from build123d import *

# Parameters (mm, degrees)
SKETCH1_W               = 79.5
SKETCH1_H               = 76
SKETCH1_R               = 4.05
BOSS_EXTRUDE1_DEPTH     = 79.5
SKETCH2_R               = 4.05
CUT_EXTRUDE1_DEPTH      = 79.5
CUT_EXTRUDE2_DEPTH      = 79.5
CUT_EXTRUDE2_DEPTH_BACK = 79.5
CUT_EXTRUDE3_DEPTH      = 79.5
CUT_EXTRUDE3_DEPTH_BACK = 79.5
SKETCH4_W               = 80.771817398
SKETCH4_H               = 76.525441438


with BuildPart() as part:
    # Sketch1 → Boss-Extrude1 (new body)
    with BuildSketch(Plane(origin=(0, 0, 0), x_dir=(1, 0, 0), z_dir=(0, 1, 0))):
        with Locations((39.75, 0)):
            Rectangle(SKETCH1_W, SKETCH1_H)
        with Locations(Location((20, 20, 0), (0, 0, 90))):
            Circle(SKETCH1_R, mode=Mode.SUBTRACT)
        with Locations(Location((60, 20, 0), (0, 0, 90))):
            Circle(SKETCH1_R, mode=Mode.SUBTRACT)
        with Locations(Location((60, -20, 0), (0, 0, 90))):
            Circle(SKETCH1_R, mode=Mode.SUBTRACT)
        with Locations(Location((20, -20, 0), (0, 0, 90))):
            Circle(SKETCH1_R, mode=Mode.SUBTRACT)
    extrude(amount=BOSS_EXTRUDE1_DEPTH)

    # Sketch2 → Cut-Extrude1 (cut)
    with BuildSketch(Plane(origin=(0, 0, 0), x_dir=(0, 0, -1), z_dir=(1, 0, 0))):
        with Locations((-20, 60)):
            Circle(SKETCH2_R)
        with Locations(Location((20, 60, 0), (0, 0, 180))):
            Circle(SKETCH2_R)
        with Locations(Location((20, 20, 0), (0, 0, 180))):
            Circle(SKETCH2_R)
        with Locations((-20, 20)):
            Circle(SKETCH2_R)
    extrude(amount=CUT_EXTRUDE1_DEPTH, mode=Mode.SUBTRACT)

    # Sketch3 → Cut-Extrude2 (cut, two sides: drawn at the far end of the back side and taken through both)
    with BuildSketch(Plane.XY.offset(-CUT_EXTRUDE2_DEPTH_BACK)):
        Polygon((4, 73.843145751), (4, 4), (73.843145751, 4), align=None)
        Polygon((4, 79.5), (79.5, 4), (79.5, 79.5), align=None)
    extrude(amount=CUT_EXTRUDE2_DEPTH + CUT_EXTRUDE2_DEPTH_BACK, mode=Mode.SUBTRACT)

    # Sketch4 → Cut-Extrude3 (cut, two sides: drawn at the far end of the back side and taken through both)
    with BuildSketch(Plane.XY.offset(-CUT_EXTRUDE3_DEPTH_BACK)):
        with Locations((44.385908699, 42.262720719)):
            Rectangle(SKETCH4_W, SKETCH4_H)
    extrude(amount=CUT_EXTRUDE3_DEPTH + CUT_EXTRUDE3_DEPTH_BACK, mode=Mode.SUBTRACT)


solid = part.part
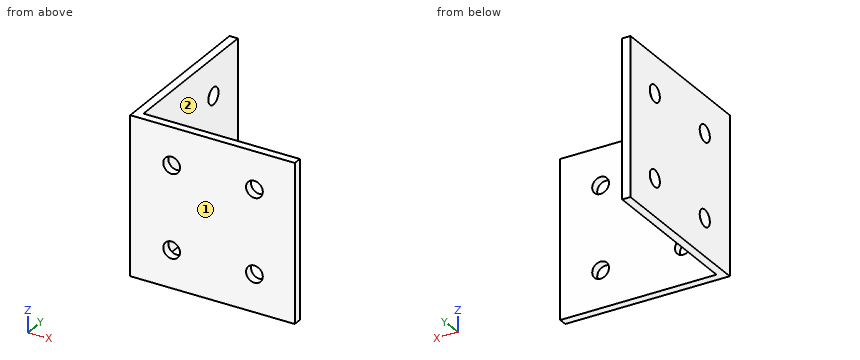
Design review of the part built by this model. Coordinates are the model's own, in mm. Face numbers are marked on the shaded views. A direction names the side the tool comes from. Give positions to 0.01 mm unless a question says otherwise; leave off trailing zeros. Order: outer loops, then holes, each group sorted by start corner. A loop starts at its lowest first (then second) coordinate and runs counter-clockwise, first axis right, second up.
1. For pin 1 Ø9.5 at (x, z) = (20, -20) entering from +Y; pin 2 Ø6.5 at (y, z) = (20, -20) entering from -X; pin 3 Ø2 at (y, z) = (42.5, -25) entering from +X; pin 4 Ø9.5 at (y, z) = (20, 20) entering from -X, all flat-tipped, find the tip position at first contact; note any pin that passes through.
Solution:
pin 1: stops at y = 4
pin 2: passes through
pin 3: stops at x = 4
pin 4: stops at x = 0
2. Add section A-A, the plane x = 60. State the section outline as (y, z) points.
Solution:
outline: (0, -38) - (4, -38) - (4, -24.05) - (0, -24.05) - close; (0, -15.95) - (4, -15.95) - (4, 15.95) - (0, 15.95) - close; (0, 24.05) - (4, 24.05) - (4, 38) - (0, 38) - close
3. Tool access review of the marked faces 1 and 2: name each direction out of +Z, -Z, +X, -X, +Y, -Y from which nothing blocks a thin tool from reaching the whole face with its end or side.
Solution:
face 1: +Z, -Z, +X, -X, -Y
face 2: +Z, -Z, +X, +Y
4. To check wall thickness, follow L1, parallel to Z at x = 1, y = 20; L2, parallel to Y at x = 2.95, z = -20. State the ranges of each line that lie inside material, in increasing order.
Solution:
L1: z = -38 to -24.05, -15.95 to 15.95, 24.05 to 38
L2: y = 0 to 15.95, 24.05 to 55.95, 64.05 to 79.5
5. Add section D-D, the plane z = 30. State the section outline as (x, y) points.
Solution:
outline: (0, 0) - (79.5, 0) - (79.5, 4) - (4, 4) - (4, 79.5) - (0, 79.5) - close
6. Add section C-C, the plane z = 20. State the section outline as (x, y) points, then the cut area to 3 significant figures.
Solution:
outline: (0, 0) - (15.95, 0) - (15.95, 4) - (4, 4) - (4, 15.95) - (0, 15.95) - close; (0, 24.05) - (4, 24.05) - (4, 55.95) - (0, 55.95) - close; (0, 64.05) - (4, 64.05) - (4, 79.5) - (0, 79.5) - close; (24.05, 0) - (55.95, 0) - (55.95, 4) - (24.05, 4) - close; (64.05, 0) - (79.5, 0) - (79.5, 4) - (64.05, 4) - close
area: 490 mm2
